Autodesk Inventor part; units mm, degrees
ref_plane "YZ Plane" through (0, 0, 0) normal (1, 0, 0) x (0, 1, 0)
ref_plane "XZ Plane" through (0, 0, 0) normal (0, 1, 0) x (-1, 0, 0)
ref_plane "XY Plane" through (0, 0, 0) normal (0, 0, 1) x (1, 0, 0)
sketch "Sketch1" plane through (0, 0, 0) normal (0, 0, 1) x (1, 0, 0)
  line L0 (-275.4313, -42) -> (-275.4313, 42)
  circle A0 centre (-243.408, 0) radius 7.5
  circle A1 centre (-130.124, 0) radius 7.5
  circle A2 centre (-50.0124, 0) radius 15.875
  circle A3 centre (-50.0124, 23.0188) radius 2.3813
  circle A4 centre (-26.9936, 0) radius 2.3813
  circle A5 centre (-73.0311, 0) radius 2.3813
  circle A6 centre (-50.0124, -23.0187) radius 2.3813
  line L1 (-275.4313, 42) -> (9.5034, 42)
  line L2 (-275.4313, -42) -> (9.5252, -42)
  line L3 (275.4312, -41.9309) -> (275.4312, 42.0691)
  line L4 (275.4312, 42.0691) -> (9.5034, 42)
  line L5 (275.4312, -41.9309) -> (9.5252, -42)
  circle A7 centre (-50.0124, 0) radius 38.1
  circle A8 centre (243.4084, 0) radius 7.5
  circle A9 centre (130.1244, 0) radius 7.5
  circle A10 centre (50.0128, 0) radius 15.875
  circle A11 centre (50.0123, 23.0188) radius 2.3813
  circle A12 centre (26.9936, 0) radius 2.3813
  circle A13 centre (73.0311, 0) radius 2.3813
  circle A14 centre (50.0123, -23.0187) radius 2.3813
  circle A15 centre (50.0128, 0) radius 38.1
  dimension "d4" = 15
  dimension "d7" = 15
  dimension "d9" = 31.75
  dimension "d11" = 4.7625
  dimension "d13" = 4.7625
  dimension "d15" = 23.0188
  dimension "d16" = 4.7625
  dimension "d18" = 4.7625
  dimension "d25" = 550.8625
  dimension "d50" = 23.0188
  dimension "d51" = 23.0188
  dimension "d52" = 23.0188
  dimension "d53" = 80.1116
  dimension "d54" = 113.284
  dimension "d62" = 76.2
  dimension "d88" = 84
  dimension "d89" = 42
  dimension "d90" = 42
  dimension "d91" = 32.0233
  dimension "d92" = 42
  dimension "d93" = 42
  dimension "d97" = 100.0252
  dimension "d98" = 80.1116
  dimension "d99" = 113.284
  dimension "d100" = 32.0228
extrude "Extrusion4" add sketch "Sketch1" along normal blind 9.525 contours L0 L1 L4 L3 L5 L2 | A7 | A15
sketch "Sketch5" plane through (0, 0, 9.525) normal (0, 0, 1) x (1, 0, 0)
  line L0 (-275.4313, -42) -> (-275.4313, 42)
  circle A0 centre (-243.408, 0) radius 7.5
  circle A1 centre (-130.124, 0) radius 7.5
  circle A2 centre (-50.0124, 0) radius 15.875
  circle A3 centre (-50.0124, 23.0188) radius 2.3813
  circle A4 centre (-26.9936, 0) radius 2.3813
  circle A5 centre (-73.0311, 0) radius 2.3813
  circle A6 centre (-50.0124, -23.0187) radius 2.3813
  line L1 (-275.4313, 42) -> (9.5034, 42)
  line L2 (-275.4313, -42) -> (9.5143, -42)
  line L3 (275.4312, -41.9309) -> (9.5143, -42)
  line L4 (275.4312, 42.0691) -> (9.5034, 42)
  line L5 (275.4312, -41.9309) -> (275.4312, 42.0691)
  circle A7 centre (-50.0124, 0) radius 38.1
  circle A8 centre (50.0123, -23.0187) radius 2.3813
  circle A9 centre (50.0123, 23.0188) radius 2.3813
  circle A10 centre (26.9936, 0) radius 2.3813
  circle A11 centre (50.0128, 0) radius 15.875
  circle A12 centre (73.0311, 0) radius 2.3813
  circle A13 centre (50.0128, 0) radius 38.1
  circle A14 centre (130.1244, 0) radius 7.5
  circle A15 centre (243.4084, 0) radius 7.5
  point P0 (0, 0)
  dimension "d103" = 15
  dimension "d104" = 15
  dimension "d105" = 31.75
  dimension "d106" = 4.7625
  dimension "d107" = 4.7625
  dimension "d108" = 23.0188
  dimension "d109" = 4.7625
  dimension "d110" = 4.7625
  dimension "d111" = 550.8625
  dimension "d112" = 23.0188
  dimension "d113" = 23.0188
  dimension "d114" = 23.0188
  dimension "d115" = 80.1116
  dimension "d116" = 113.284
  dimension "d117" = 76.2
  dimension "d118" = 84
  dimension "d119" = 42
  dimension "d120" = 42
  dimension "d121" = 32.0233
  dimension "d122" = 42
  dimension "d123" = 42
  dimension "d124" = 100.0252
  dimension "d125" = 80.1116
  dimension "d126" = 113.284
  dimension "d127" = 32.0228
emboss "Emboss4" sketch "Sketch5" operation cut depth 3 direction (0, 0, -1) contours A7 | A13
properties part number "Drivetrainsideinside"
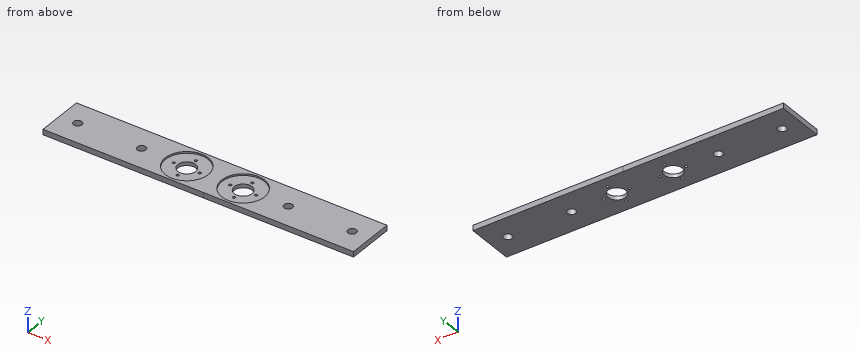
Geometry check sheet. Reference: the model listing, model coordinates, mm. Coordinates: 2 decimals unless noted, no trailing zeros. Order: outer loops, then holes, each group sorted by start corner. A loop starts at its lowest first (then second) coordinate and runs counter-clockwise, first axis right, second up.
Item 1: Section check B-B (y = -30). Enter the section's corners in (x, z) (3 decimals), plus the area to 3 significant figures.
Item 2: Section check A-A (z = 8). Enter the section's corners in (x, y).
Item 3: Depth check by flat-ended pin: pin 1 (4 mm diameter, centred on x = 73.03, y = 0, fed in from -Z); pin 2 (1 mm diameter, centred on x = -78.5, y = -15.5, fed in from -Z); pin 3 (5 mm diameter, centred on x = 133.5, z = 5.5, fed in from +Y); pin 4 (7.5 mm diameter, centred on x = 26.99, y = 0, fed in from +Z) (3 decimals). Enter the tip coordinate at first touch or a pass-through.
Item 4: Scan lines: line 1 along X through (y, z) = (29, 9); line 2 along Y through (x, z) = (149, 7.5); line 3 along X through (y, z) = (24.5, 5). Record each from-to range of solid material in increasing order.
Check sheet entries:
1. outline: (-275.431, 0) - (275.431, 0) - (275.431, 9.525) - (73.499, 9.525) - (73.499, 6.525) - (26.526, 6.525) - (26.526, 9.525) - (-26.526, 9.525) - (-26.526, 6.525) - (-73.499, 6.525) - (-73.499, 9.525) - (-275.431, 9.525) - close
1. area: 4,970 mm2
2. outline: (-275.43, -42) - (9.53, -42) - (275.43, -41.93) - (275.43, 42.07) - (9.5, 42) - (-275.43, 42) - close; hole circle Ø15 at (-243.41, 0); hole circle Ø15 at (-130.12, 0); hole circle Ø76.2 at (-50.01, 0); hole circle Ø76.2 at (50.01, 0); hole circle Ø15 at (130.12, 0); hole circle Ø15 at (243.41, 0)
3. pin 1: passes through
3. pin 2: stops at z = 0
3. pin 3: stops at y = 42.03
3. pin 4: stops at z = 6.525
4. line 1: x = -275.43 to -74.72, -25.3 to 25.3, 74.72 to 275.43
4. line 2: y = -41.96 to 42.04
4. line 3: x = -275.43 to -51.88, -48.15 to 48.15, 51.88 to 275.43
